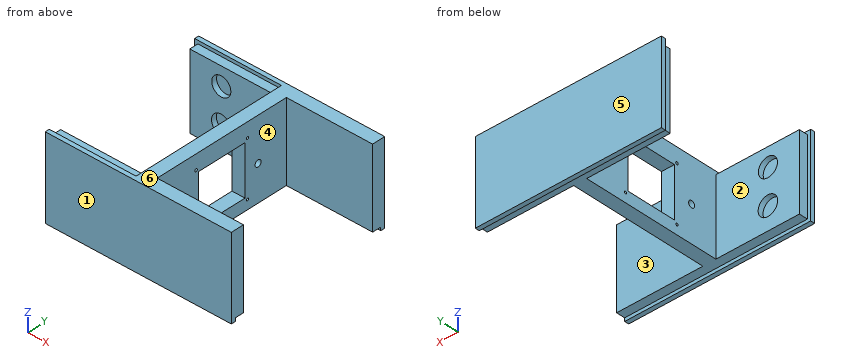
Solid Edge part; units mm, degrees
sketch "Sketch1" plane through (0, 0, 0) normal (0, -1, 0) x (1, 0, 0)
  line L0 (-136.525, 69.85) -> (135.763, 69.85)
  line L1 (135.763, 69.85) -> (135.763, -50.8)
  line L2 (135.763, -50.8) -> (-136.525, -50.8)
  line L3 (-136.525, -50.8) -> (-136.525, 69.85)
  dimension "D1" = 136.525
  dimension "D2" = 136.525
extrude "Protrusion1" add sketch "Sketch1" along normal mid plane 241.3
sketch "Sketch2" plane through (0, 0, 0) normal (1, 0, 0) x (0, 1, 0)
  line L0 (101.6, -69.85) -> (-101.6, -69.85)
  line L1 (-101.6, -69.85) -> (-101.6, 69.85)
  line L2 (-101.6, 69.85) -> (101.6, 69.85)
  line L3 (101.6, 69.85) -> (101.6, -69.85)
extrude "Cutout1" cut sketch "Sketch2" along normal up to next and the other way up to next
sketch "Sketch3" plane through (6.4194, -101.6, 0) normal (0, 1, 0) x (-1, 0, 0)
  line L0 (138.1819, -46.0375) -> (15.9444, -46.0375)
  line L1 (15.9444, -50.8) -> (15.9444, -46.0375)
  line L2 (15.9444, -50.8) -> (142.9444, -50.8)
  line L3 (142.9444, -50.8) -> (142.9444, 69.85)
  line L4 (142.9444, 69.85) -> (15.9444, 69.85)
  line L5 (15.9444, 65.0875) -> (15.9444, 69.85)
  line L6 (15.9444, 65.0875) -> (138.1819, 65.0875)
  line L7 (138.1819, 65.0875) -> (138.1819, -46.0375)
extrude "ExtrudedCutout_2" cut sketch "Sketch3" against normal blind 12.7
mirror "Mirror1" about plane through (0, 0, 0) normal (0, 1, 0) of "ExtrudedCutout_2"
sketch "Sketch4" plane through (21.4313, 101.6, 12.7) normal (0, -1, 0) x (1, 0, 0)
  circle A0 centre (-107.1563, -25.4) radius 14.2875
  circle A1 centre (-107.1563, 25.4) radius 13.97
extrude "ExtrudedCutout_3" cut sketch "Sketch4" against normal blind 7.62
mirror "Mirror2" about plane through (0, 0, 0) normal (0, -1, 0) of "ExtrudedCutout_3"
sketch "Sketch5" plane through (6.4194, 0, 0) normal (0, -1, 0) x (1, 0, 0)
  line L0 (-15.9444, -46.0375) -> (3.1056, -46.0375)
  line L1 (3.1056, -46.0375) -> (3.1056, 69.85)
  line L2 (3.1056, 69.85) -> (-15.9444, 69.85)
  line L3 (-15.9444, 69.85) -> (-15.9444, -46.0375)
  dimension "D1" = 15.9444
extrude "Protrusion2" add sketch "Sketch5" along normal up to next and the other way up to next
sketch "Sketch6" plane through (0, 0, 0) normal (1, 0, 0) x (0, 1, 0)
  line L0 (36.5125, -28.575) -> (-36.5125, -28.575)
  line L1 (-36.5125, -28.575) -> (-36.5125, 44.45)
  line L2 (-36.5125, 44.45) -> (36.5125, 44.45)
  line L3 (36.5125, 44.45) -> (36.5125, -28.575)
  circle A0 centre (-40.4813, 48.4187) radius 1.9984
  circle A1 centre (-40.4812, -32.5438) radius 1.7985
  circle A2 centre (40.4813, 48.4187) radius 1.7985
  circle A3 centre (40.4813, -32.5438) radius 1.7985
  dimension "D1" = 36.5125
  dimension "D2" = 36.5125
extrude "Cutout2" cut sketch "Sketch6" along normal up to next and the other way up to next
sketch "Sketch7" plane through (-9.525, 0, 3.175) normal (-1, 0, 0) x (0, -1, 0)
  circle A0 centre (-57.15, 3.175) radius 4.7625
  circle A1 centre (63.5, 3.175) radius 4.7625
extrude "Cutout3" cut sketch "Sketch7" against normal up to next
sketch "Sketch8" plane through (-136.525, 117.475, 0) normal (-1, 0, 0) x (0, 0, 1)
  line L0 (-46.0375, -3.175) -> (-50.8, -3.175)
  line L1 (-50.8, -3.175) -> (-50.8, -15.875)
  line L2 (-50.8, -15.875) -> (-46.0375, -15.875)
  line L3 (-46.0375, -15.875) -> (-46.0375, -3.175)
extrude "Cutout4" cut sketch "Sketch8" against normal up to next
mirror "Mirror3" about plane through (0, 0, 0) normal (0, -1, 0) of "Cutout4"
Geometry: final body of the model. Coordinates: model frame, mm. Face numbers are marked on the shaded views. A direction names the side the tool comes from. Give positions to 0.01 mm unless a question says otherwise; leave off trailing zeros. Order: outer loops, then holes, each group sorted by start corner. A loop starts at its lowest first (then second) coordinate and runs counter-clockwise, first axis right, second up. Notation, with made-up numbers: (-21.75, -18) - (12.25, -18) arc R34 ccw to (12.25, 18) - close; hole circle Ø10 at (75, 24). An arc over 180 degrees is marked (long way). Use CSV: the item, a comma, the result in double quotes.
1. Mould query, pull axis Y, two halves, no side actions, for the marked faces 4, 5 and 6. Classes: +Y half, -Y half, draft (parallel to the pull), parting line (faces both ways), or undercut.
Answers below:
face 4,"undercut"
face 5,"+Y half"
face 6,"draft"
2. Contact query for flat-ended pins moving along their axis: pin 1 (12 mm diameter, centred on x = 87, y = -90.5, fed in from -Z); pin 2 (4.5 mm diameter, centred on y = 40.48, z = -32.54, fed in from -X) (3 decimals); pin 3 (10 mm diameter, centred on y = -105.5, z = 8.5, fed in from -X); pin 4 (4 mm diameter, centred on x = -98.5, y = -107, fed in from +Z). Output: stop coordinate, or through.
Answers below:
pin 1,"through"
pin 2,"x = -9.525"
pin 3,"x = -131.76"
pin 4,"z = 65.09"
3. Section query A-A (x = 108.5). Output: boundary loops of the cut face in (y, z).
Answers below:
outline,"(-120.65, -50.8) - (-114.3, -50.8) - (-114.3, -46.04) - (-101.6, -46.04) - (-101.6, 69.85) - (-120.65, 69.85) - close; (101.6, -46.04) - (114.3, -46.04) - (114.3, -50.8) - (120.65, -50.8) - (120.65, 69.85) - (101.6, 69.85) - close"
4. Material intervals for line 1 along Y through (x, z) = (66, 2.5); line 2 along X through (y, z) = (-73, 47) (3 decimals); line 3 along X through (y, z) = (-106, 33.5), sorted ascending. Write a range as from..to.
Answers below:
line 1,"-120.65..-101.6, 101.6..120.65"
line 2,"-9.525..9.525"
line 3,"-131.76..-98.92, -72.53..135.76"
5. Section query D-D (z = 6.35). Give the number of separate pieces and of enclosed holes in the cut face, plus the area to 3 significant figures.
Answers below:
separate pieces,"4"
enclosed holes,"0"
area,"12,400 mm2"
6. Access query for the marked faces 1, 2 and 3. Directions: +Z, -Z, +X, -X, +Y, -Y. A direction counts if a zero-diameter tool reaches every point of the face in a straight line with its end or side. Return the directions, or none.
Answers below:
face 1,"+Z, -Z, +X, -X, -Y"
face 2,"+Z, -Z, -X"
face 3,"+Z, -Z, +X"
